Could you check a few things on this model? Use its own coordinates, in mm. Coordinates: 2 decimals unless noted, no trailing zeros. Order: outer loops, then holes, each group sorted by start corner. A loop starts at its lowest first (then second) coordinate and runs counter-clockwise, first axis right, second up. Notation, with made-up numbers: (15, 60.25) - (28, 60.25) arc R22 ccw to (28, 89.25) - close; hole circle Ø6 at (-32, 78.5). An arc over 180 degrees is marked (long way). Answer as CSV lines item,"result". Start each with the question number.
1. I want a section at B-B, the plane x = 13. List the corners of the cut face in (y, z) for me, and give its area (3 significant figures).
2. I want a section at D-D, the plane x = 0. List the corners of the cut face in (y, z) for me, and give its area (3 significant figures).
3. I want a section at C-C, the plane y = 8. List the corners of the cut face in (x, z) for me, and give its area (3 significant figures).
4. I want a section at A-A, the plane z = -0.5. List the corners of the cut face in (x, y) for me (3 decimals), and give its area (3 significant figures).
5. For pin 1 (1 mm diameter, centred on x = 19.5, y = 23, fed in from -Z); pin 2 (20 mm diameter, centred on x = 8, z = -2.5, fed in from -Y), each with a flat end and sliding along its axis, tell me the tip position at first contact or that it passes through.
6. I need wall thicknesses on probe 1 along Y at (x, z) = (-5.5, 30); probe 2 along X at (y, z) = (54, 32.5); probe 3 along Z at (x, y) = (-9, 90.5). Which ranges of each line are inside material? Lowest first, please.
from build123d import *

# Parameters (mm, degrees)
SKETCH3_W           = 59.69
SKETCH3_H           = 84.074
BOSS_EXTRUDE1_DEPTH = 93.98
SKETCH4_W           = 59.69
SKETCH4_H           = 84.074
SKETCH4_R           = 5.08
CUT_EXTRUDE1_DEPTH  = 20
FILLET1_R           = 10


with BuildPart() as part:
    # Sketch3 → Boss-Extrude1 (new body)
    with BuildSketch(Plane(origin=(0, 0, 0), x_dir=(1, 0, 0), z_dir=(0, 1, 0))):
        Rectangle(SKETCH3_W, SKETCH3_H)
    extrude(amount=BOSS_EXTRUDE1_DEPTH)

    # Sketch4 → Cut-Extrude1 (cut)
    with BuildSketch(Plane.XZ):
        Rectangle(SKETCH4_W, SKETCH4_H)
        with Locations((0, 25.4)):
            Circle(SKETCH4_R, mode=Mode.SUBTRACT)
    extrude(amount=-CUT_EXTRUDE1_DEPTH, mode=Mode.SUBTRACT)

    # Fillet1
    fillet1_edges = [part.edges().sort_by_distance(p)[0] for p in [
        (-29.845, 93.98, 0),
        (0, 93.98, 42.037),
        (0, 20, -42.037),
        (-29.845, 20, 0),
        (0, 20, 42.037),
        (29.845, 20, 0),
        (29.845, 93.98, 0),
        (0, 93.98, -42.037),
        (29.845, 56.99, 42.037),
        (-29.845, 56.99, 42.037),
        (-29.845, 56.99, -42.037),
        (29.845, 56.99, -42.037),
    ]]
    fillet(fillet1_edges, radius=FILLET1_R)


solid = part.part
Solved:
1,outline,"(20, -32.04) arc R10 ccw to (30, -42.04) - (83.98, -42.04) arc R10 ccw to (93.98, -32.04) - (93.98, 32.04) arc R10 ccw to (83.98, 42.04) - (30, 42.04) arc R10 ccw to (20, 32.04) - close"
1,area,"6,130 mm2"
2,outline,"(0, 20.32) - (20, 20.32) - (20, -32.04) arc R10 ccw to (30, -42.04) - (83.98, -42.04) arc R10 ccw to (93.98, -32.04) - (93.98, 32.04) arc R10 ccw to (83.98, 42.04) - (30, 42.04) arc R10 ccw to (20, 32.04) - (20, 30.48) - (0, 30.48) - close"
2,area,"6,340 mm2"
3,outline,"circle Ø10.16 at (0, 25.4)"
3,area,"81.1 mm2"
4,outline,"(-29.845, 30) arc R10 ccw to (-19.845, 20) - (19.845, 20) arc R10 ccw to (29.845, 30) - (29.845, 83.98) arc R10 ccw to (19.845, 93.98) - (-19.845, 93.98) arc R10 ccw to (-29.845, 83.98) - close"
4,area,"4,330 mm2"
5,pin 1,"stops at z = -39.64"
5,pin 2,"stops at y = 20"
6,probe 1,"y = 20 to 93.98"
6,probe 2,"x = -29.83 to 29.83"
6,probe 3,"z = -39.62 to 39.62"
